Geometry: see drawing. Coordinates: mm, zero at the bounding-box minimum. A direction names the side the tool comes from. Round coordinates to 2 decimals unless told otherwise and drop trailing zeros. Order: outer loops, then holes, each group sorted by start corner. A loop starts at its lowest first (then second) coordinate and runs counter-clockwise, first axis right, second up. Notation, with made-up numbers: (70.25, 11) -> (90.25, 11) arc R16 cw to (90.25, 20) -> close; hole circle Ø1 at (-18.5, -29). An arc over 180 degrees is marked (long way). Answer as CSV lines item,"result". Start each with the question number.
(1) Set-up query: the marked faces 5, 6 and 7. Return all of +Z, -Z, +X, -X, +Y, -Y with unobstructed straight access to the full face (end or side cutting, diameter ignored); none if empty.
(2) Section query A-A (z = 7.5). Output: boundary loops of the cut face in (x, y).
(3) Section query B-B (x = 102.5). Output: boundary loops of the cut face in (y, z), plus the area to 3 significant figures.
(4) Pull-direction query (Y, two-part tool) for the marked faces 1, 2, 3 and 4; classes: +Y half, -Y half, draft (parallel to the pull), parting line (faces both ways), or undercut.
(5) Line query: line 1 along Y through (x, z) = (35, 21.5); line 2 along Y through (x, z) = (75, 8); line 3 along X through (y, z) = (12.5, 4.5). Output: solid intervals per line, ascending. Write a range as from..to.
(6) Contact query for flat-ended pins moving along their axis: P1, Ø6.5, axis at x = 74, y = 49, coming from the +Z side; P2, Ø10.5, axis at x = 38, y = 47, coming from the +Z side (1 decimal); P3, Ø6, axis at x = 104.5, y = 29.5, coming from the -Z side; P4, Ø3.5, axis at x = 102.5, y = 10, coming from the +Z side. Output: stop coordinate, or through.
(7) Section query D-D (y = 24.5). Output: boundary loops of the cut face in (x, z), plus the area to 3 significant figures.
(8) Section query C-C (z = 36). Output: boundary loops of the cut face in (x, y).
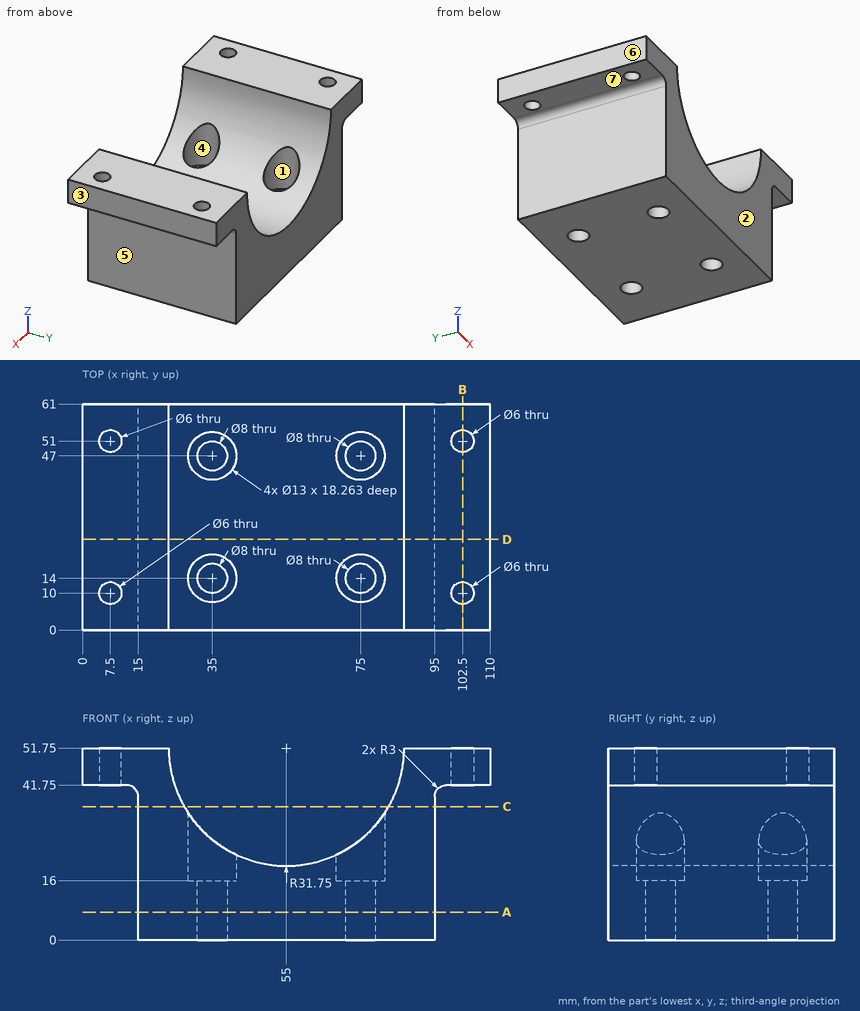
Answer block:
1,face 5,"-Z, +X, +Y, -Y"
1,face 6,"+Z, -Z, -X, +Y, -Y"
1,face 7,"-Z, -X, +Y, -Y"
2,outline,"(15, 0) -> (95, 0) -> (95, 61) -> (15, 61) -> close; hole circle Ø8 at (35, 14); hole circle Ø8 at (35, 47); hole circle Ø8 at (75, 14); hole circle Ø8 at (75, 47)"
3,outline,"(0, 41.75) -> (7, 41.75) -> (7, 51.75) -> (0, 51.75) -> close; (13, 41.75) -> (48, 41.75) -> (48, 51.75) -> (13, 51.75) -> close; (54, 41.75) -> (61, 41.75) -> (61, 51.75) -> (54, 51.75) -> close"
3,area,"490 mm2"
4,face 1,"undercut"
4,face 2,"-Y half"
4,face 3,"draft"
4,face 4,"undercut"
5,line 1,"0..7.5, 20.5..40.5, 53.5..61"
5,line 2,"0..10, 18..43, 51..61"
5,line 3,"15..31.29, 38.71..71.29, 78.71..95"
6,P1,"z = 16"
6,P2,"z = 24.4"
6,P3,"z = 41.75"
6,P4,"through"
7,outline,"(0, 41.75) -> (12, 41.75) arc R3 cw to (15, 38.75) -> (15, 0) -> (95, 0) -> (95, 38.75) arc R3 cw to (98, 41.75) -> (110, 41.75) -> (110, 51.75) -> (86.75, 51.75) arc R31.75 cw to (23.25, 51.75) -> (0, 51.75) -> close"
7,area,"2,860 mm2"
8,outline,"(15, 0) -> (27.43, 0) -> (27.43, 61) -> (15, 61) -> close; (82.57, 0) -> (95, 0) -> (95, 61) -> (82.57, 61) -> close"
